from build123d import *

# Parameters (mm, degrees)
SKETCH_1_R          = 1.65
EXTRUDE_1_DEPTH     = 8
FILLET_1_R          = 10
SKETCH_2_R          = 4
CUT_EXTRUDE_1_DEPTH = 3


with BuildPart() as part:
    # 草圖1 → 填料-伸長1 (new body)
    with BuildSketch(Plane.XY):
        with BuildLine():
            Line((0, -5), (22.896270517, -5))
            ThreePointArc((22.896270517, -5), (63.449308727, 34.693340668), (47.334627368, 89.103149031))
            Line((47.334627368, 89.103149031), (39.525260877, 67.647090937))
            ThreePointArc((39.525260877, 67.647090937), (38.24035653, 27.551768918), (0.138664652, 15))
            Line((0.138664652, 15), (-4.698463104, 1.710100717))
            ThreePointArc((-4.698463104, 1.710100717), (-4.095760221, -2.867882182), (0, -5))
        make_face()
        Circle(SKETCH_1_R, mode=Mode.SUBTRACT)
        with Locations((16.5, 0)):
            Circle(SKETCH_1_R, mode=Mode.SUBTRACT)
    extrude(amount=EXTRUDE_1_DEPTH)

    # 圓角1
    fillet_1_edges = [part.edges().sort_by_distance(p)[0] for p in [
        (0.138664652, 15, 4),
    ]]
    fillet(fillet_1_edges, radius=FILLET_1_R)

    # 草圖2 → 除料-伸長1 (cut)
    with BuildSketch(Plane(origin=(0, 0, 0), x_dir=(-1, 0, 0), z_dir=(0, 0, -1))):
        Circle(SKETCH_2_R)
    extrude(amount=-CUT_EXTRUDE_1_DEPTH, mode=Mode.SUBTRACT)


solid = part.part
Verification items for the finished model (mm, model axes). A direction names the side the tool comes from. Coordinates: 2 decimals unless noted, no trailing zeros. Write each loop counter-clockwise with the first axis right and the second up, starting at its lowest first coordinate (ties: lowest second). Pieces come first, ordered by that corner, then holes. Notation, with made-up numbers: (-18, -18.5) - (13, -18.5) arc R20 ccw to (13, 0.5) - close; hole circle Ø9 at (-23, 66.25). An arc over 180 degrees is marked (long way). Answer as a JSON object with one key per item and string values.
(1) Mould release check, pull along X, two halves, no side actions. Record for faces 3 (the flat face through (-2, 0, 3)), 4 (the cylindrical face through (63.233, 33.887, 3.944)), 5 (the flat face through (-3.71, 4.43, 3.94)): pulls with the +X half, pulls with the -X half, needs draft (parallel to the pull), parting line crosses it, or undercut.
Report:
{"face 3": "undercut", "face 4": "pulls with the +X half", "face 5": "pulls with the -X half"}
(2) Tool access check on faces 1 (the cylindrical face through (18.074, 0.496, 3.944)), 2 (the cylindrical face through (0.867, -3.905, 1.479)). Record the directions out of +Z, -Z, +X, -X, +Y, -Y that give a thin tool (end or side, any length) a straight path to the whole face; none if there is none.
Report:
{"face 1": "+Z, -Z", "face 2": "-Z"}
(3) Cross-section at B-B on y = 0. Record the cut outline in (x, z).
Report:
{"outline": "(-5, 0) - (-4, 0) - (-4, 3) - (-1.65, 3) - (-1.65, 8) - (-5, 8) - close; (1.65, 3) - (4, 3) - (4, 0) - (14.85, 0) - (14.85, 8) - (1.65, 8) - close; (18.15, 0) - (36.12, 0) - (36.12, 8) - (18.15, 8) - close"}
(4) Thickness scan on line 1 along X through (y, z) = (0.5, 2); line 2 along Y through (x, z) = (16.5, 3.25); line 3 along X through (y, z) = (32, 7.25). Record the ranges inside material, lowest first.
Report:
{"line 1": "-4.97 to -3.97, 3.97 to 14.93, 18.07 to 37.03", "line 2": "-5 to -1.65, 1.65 to 14.09", "line 3": "41.07 to 62.68"}
(5) Cross-section at C-C on x = 16.5. Record the cut outline in (y, z), plus the area to 3 significant figures.
Report:
{"outline": "(-5, 0) - (-1.65, 0) - (-1.65, 8) - (-5, 8) - close; (1.65, 0) - (14.09, 0) - (14.09, 8) - (1.65, 8) - close", "area": "126 mm^2"}
(6) Gauge pin test, flat ends, axial feed: pin 1 Ø1 at (x, z) = (17.5, 1.5) entering from +Y; pin 2 Ø3 at (x, z) = (57, 6) entering from +Y; pin 3 Ø4 at (x, y) = (0, -0.5) entering from -Z; pin 4 Ø3 at (x, y) = (0, 0) entering from +Z. Record the tip position at first contact, or that the pin passes through.
Report:
{"pin 1": "y = 14.39", "pin 2": "y = 79.73", "pin 3": "z = 3", "pin 4": "through"}
(7) Cross-section at D-D on y = 80.5. Record the cut outline in (x, z).
Report:
{"outline": "(44.2, 0) - (54.96, 0) - (54.96, 8) - (44.2, 8) - close"}
(8) Cross-section at A-A on z = 6.25. Record the cut outline in (x, y).
Report:
{"outline": "(-4.7, 1.71) arc R5 ccw to (0, -5) - (22.9, -5) arc R55 ccw to (47.33, 89.1) - (39.53, 67.65) arc R35 cw to (7.44, 13.63) arc R10 ccw to (-2.74, 7.08) - close; hole circle Ø3.3 at (0, 0); hole circle Ø3.3 at (16.5, 0)"}
